Check sheet for the modelled part. Datum: model origin and axes. Units: mm. Face numbers are marked on the shaded views. Coordinates: 2 decimals unless noted, no trailing zeros. Loops run counter-clockwise (first coordinate to the right, second up) from the corner with the lowest first, then second, coordinate; pieces in that order, holes last. Notation, with made-up numbers: (23.5, 82) -> (59.5, 82) arc R12 cw to (59.5, 102) -> close; hole circle Ø2 at (16.25, 64). An arc over 180 degrees is marked (long way). Use CSV: the item, a comma, the result in double quotes.
```python
from build123d import *

# Parameters (mm, degrees)
F0_W      = 228.6
F0_H      = 228.6
F1_DEPTH  = 12.7
F2_W      = 152.4
F2_H      = 215.9
F3_DEPTH  = 76.2
F4_DEPTH  = 63.5
F5_R      = 9.525
F6_DEPTH  = 12.7
F7_R      = 9.525
F8_DEPTH  = 82.55
F9_W      = 38.1
F9_H      = 101.6
F10_DEPTH = 15.875
F11_W     = 3.175
F11_H     = 101.6
F12_DEPTH = 50.8
F13_R     = 2.54
F14_R     = 7.62


with BuildPart() as f1:
    # F0 (on Top) → F1 (new body)
    with BuildSketch(Plane.XY):
        Rectangle(F0_W, F0_H)
    extrude(amount=F1_DEPTH)

    # F2 (on Right) → F3 (join, symmetric)
    with BuildSketch(Plane.YZ):
        with Locations((0, 120.65)):
            Rectangle(F2_W, F2_H)
    extrude(amount=F3_DEPTH, both=True)

    # F2 (on Right) → F4 (cut, symmetric)
    with BuildSketch(Plane.YZ):
        with Locations((0, 120.65)):
            Rectangle(F2_W, F2_H)
    extrude(amount=F4_DEPTH, both=True, mode=Mode.SUBTRACT)

    # F5 (on Top) → F6 (cut, symmetric)
    with BuildSketch(Plane.XY):
        Circle(F5_R)
    extrude(amount=F6_DEPTH, both=True, mode=Mode.SUBTRACT)

    # F7 (on Right) → F8 (join, symmetric)
    with BuildSketch(Plane.YZ):
        with Locations((50.8, 88.9)):
            Circle(F7_R)
    extrude(amount=F8_DEPTH, both=True)

    # F9 (on Top) → F10 (join)
    with BuildSketch(Plane.XY):
        with Locations((-95.25, 0)):
            Rectangle(F9_W, F9_H)
        with Locations((95.25, 0)):
            Rectangle(F9_W, F9_H)
    extrude(amount=F10_DEPTH)

    # F11 (on Top) → F12 (join)
    with BuildSketch(Plane.XY):
        with Locations((-77.7875, 0)):
            Rectangle(F11_W, F11_H)
        with Locations((77.7875, 0)):
            Rectangle(F11_W, F11_H)
    extrude(amount=F12_DEPTH)

    # F13
    f13_edges = [f1.edges().sort_by_distance(p)[0] for p in [
        (-114.3, 0, 15.875),
        (-79.375, 0, 50.8),
        (79.375, 0, 50.8),
        (114.3, 0, 15.875),
    ]]
    fillet(f13_edges, radius=F13_R)

    # F14
    f14_edges = [f1.edges().sort_by_distance(p)[0] for p in [
        (-79.375, 0, 15.875),
        (79.375, 0, 15.875),
    ]]
    fillet(f14_edges, radius=F14_R)


solid = f1.part
```
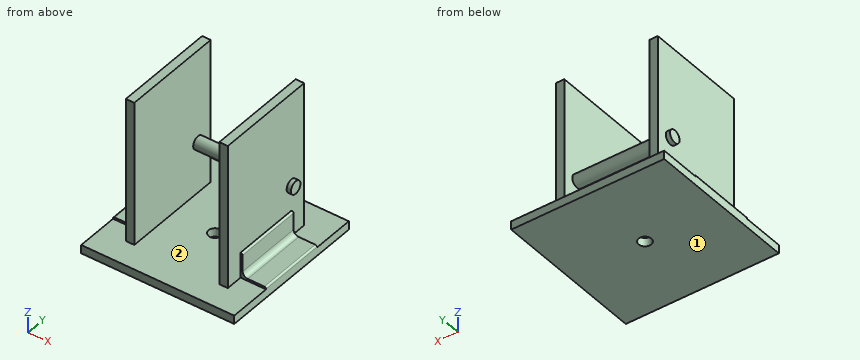
1) Go/stop test with flat-tipped pins: pin 1 Ø21 at (y, z) = (54, 87.5) entering from +X; pin 2 Ø8 at (y, z) = (-16, 125) entering from +X; pin 3 Ø12.5 at (x, y) = (95.5, 15) entering from +Z (3 decimals). Record where each tip stops, or that it passes through.
Answer below:
pin 1,"stops at x = 82.55"
pin 2,"stops at x = 76.2"
pin 3,"stops at z = 15.875"
2) Thickness scan on line 1 along X through (y, z) = (51, 184); line 2 along Y through (x, z) = (0, 4) (3 decimals); line 3 along Z through (x, y) = (-31.5, -24). Record the ranges inside material, lowest first. Write a range as from..to.
Answer below:
line 1,"x = -76.2..-63.5, 63.5..76.2"
line 2,"y = -114.3..-9.525, 9.525..114.3"
line 3,"z = 0..12.7"
3) Cross-section at B-B on x = 0. Record the boundary of the cut face in (y, z) (3 decimals).
Answer below:
outline,"(-114.3, 0) -> (-9.525, 0) -> (-9.525, 12.7) -> (-114.3, 12.7) -> close; (9.525, 0) -> (114.3, 0) -> (114.3, 12.7) -> (9.525, 12.7) -> close; circle Ø19.05 at (50.8, 88.9)"
4) Cross-section at D-D on y = 36.5. Record the boundary of the cut face in (x, z) (3 decimals).
Answer below:
outline,"(-114.3, 0) -> (114.3, 0) -> (114.3, 13.335) arc R2.54 ccw to (111.76, 15.875) -> (86.995, 15.875) arc R7.62 cw to (79.375, 23.495) -> (79.375, 48.26) arc R2.54 ccw to (76.835, 50.8) -> (76.2, 50.8) -> (76.2, 228.6) -> (63.5, 228.6) -> (63.5, 12.7) -> (-63.5, 12.7) -> (-63.5, 228.6) -> (-76.2, 228.6) -> (-76.2, 50.8) -> (-76.835, 50.8) arc R2.54 ccw to (-79.375, 48.26) -> (-79.375, 23.495) arc R7.62 cw to (-86.995, 15.875) -> (-111.76, 15.875) arc R2.54 ccw to (-114.3, 13.335) -> close"
5) Cross-section at C-C on z = 214. Record the boundary of the cut face in (x, y), and give its area (3 significant figures).
Answer below:
outline,"(-76.2, -76.2) -> (-63.5, -76.2) -> (-63.5, 76.2) -> (-76.2, 76.2) -> close; (63.5, -76.2) -> (76.2, -76.2) -> (76.2, 76.2) -> (63.5, 76.2) -> close"
area,"3,870 mm²"
6) Cross-section at A-A on y = 0. Record the boundary of the cut face in (x, z) (3 decimals), and give its area (3 significant figures).
Answer below:
outline,"(-114.3, 0) -> (-9.525, 0) -> (-9.525, 12.7) -> (-63.5, 12.7) -> (-63.5, 228.6) -> (-76.2, 228.6) -> (-76.2, 50.8) -> (-76.835, 50.8) arc R2.54 ccw to (-79.375, 48.26) -> (-79.375, 23.495) arc R7.62 cw to (-86.995, 15.875) -> (-111.76, 15.875) arc R2.54 ccw to (-114.3, 13.335) -> close; (9.525, 0) -> (114.3, 0) -> (114.3, 13.335) arc R2.54 ccw to (111.76, 15.875) -> (86.995, 15.875) arc R7.62 cw to (79.375, 23.495) -> (79.375, 48.26) arc R2.54 ccw to (76.835, 50.8) -> (76.2, 50.8) -> (76.2, 228.6) -> (63.5, 228.6) -> (63.5, 12.7) -> (9.525, 12.7) -> close"
area,"8,630 mm²"
7) Draft check along X on the marked faces 1 and 2. Enter one of: released by +X, released by -X, zero draft, split by the parting line, or undercut.
Answer below:
face 1,"zero draft"
face 2,"undercut"
